from build123d import *

# Parameters (mm, degrees)
SKETCH1_R           = 20
SKETCH1_R_2         = 12
SKETCH1_R_3         = 2.5
SKETCH1_R_4         = 10
BOSS_EXTRUDE1_DEPTH = 3
BOSS_EXTRUDE2_START = 10
SKETCH1_3_R         = 12
SKETCH1_3_R_2       = 10
BOSS_EXTRUDE2_DEPTH = 10


with BuildPart() as part:
    # Sketch1 → Boss-Extrude1 (new body)
    # profile 1 of 2: a face of its own
    with BuildSketch(Plane(origin=(0, 0, 0), x_dir=(1, 0, 0), z_dir=(0, 1, 0))):
        with Locations(Location((0, 0, 0), (0, 0, 270))):
            Circle(SKETCH1_R)
        Circle(SKETCH1_R_2, mode=Mode.SUBTRACT)
        with Locations(Location((-12.990381057, -7.5, 0), (0, 0, 270))):
            Circle(SKETCH1_R_3, mode=Mode.SUBTRACT)
        with Locations(Location((12.990381057, -7.5, 0), (0, 0, 270))):
            Circle(SKETCH1_R_3, mode=Mode.SUBTRACT)
        with Locations(Location((0, 15, 0), (0, 0, 270))):
            Circle(SKETCH1_R_3, mode=Mode.SUBTRACT)
    # profile 2 of 2: a face of its own
    with BuildSketch(Plane(origin=(0, 0, 0), x_dir=(1, 0, 0), z_dir=(0, 1, 0))):
        Circle(SKETCH1_R_2)
        with Locations(Location((0, 0, 0), (0, 0, 270))):
            Circle(SKETCH1_R_4, mode=Mode.SUBTRACT)
    extrude(amount=-BOSS_EXTRUDE1_DEPTH)

    # Sketch1_3 → Boss-Extrude2 (add)
    with BuildSketch(Plane(origin=(0, 0, 0), x_dir=(1, 0, 0), z_dir=(0, 1, 0)).offset(BOSS_EXTRUDE2_START)):
        with Locations(Location((0, 0, 0), (0, 0, 270))):
            Circle(SKETCH1_3_R)
        with Locations(Location((0, 0, 0), (0, 0, 270))):
            Circle(SKETCH1_3_R_2, mode=Mode.SUBTRACT)
    extrude(amount=-BOSS_EXTRUDE2_DEPTH)


solid = part.part
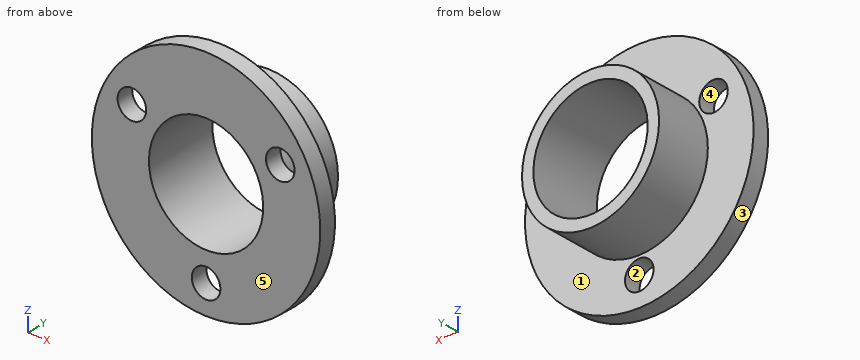
For this review, take the finished solid that the model builds, in its own axes (mm). Face numbers are marked on the shaded views. A direction names the side the tool comes from. Coordinates: 2 decimals unless noted, no trailing zeros. Loops run counter-clockwise (first coordinate to the right, second up) from the corner with the lowest first, then second, coordinate; pieces in that order, holes last. Notation, with made-up numbers: (69, -1) - (93, -1) arc R21 cw to (93, 18) - close; hole circle Ø10 at (79.25, 54). An arc over 180 degrees is marked (long way). Return JSON: item names as keys, results as strings.
Item 1: Mouldability with a two-part tool opening along Z and no side actions: class the marked faces 3, 4 and 5 as pulls with the +Z half, pulls with the -Z half, needs draft (parallel to the pull), parting line crosses it, or undercut.
Determined:
{"face 3": "parting line crosses it", "face 4": "undercut", "face 5": "needs draft"}
Item 2: For the marked faces 1 and 2, list the 3-axis set-ups (+Z, -Z, +X, -X, +Y, -Y) from which the entire face can be reached by the end or side of a thin tool; tool diameter is ignored.
Determined:
{"face 1": "+Y", "face 2": "+Y, -Y"}
Item 3: Take a section at B-B (z = 0). Give the boundary of the cut face in (x, y), then the cut area to 3 significant figures.
Determined:
{"outline": "(-20, -3) - (-10, -3) - (-10, 10) - (-12, 10) - (-12, 0) - (-20, 0) - close; (10, -3) - (20, -3) - (20, 0) - (12, 0) - (12, 10) - (10, 10) - close", "area": "100 mm2"}
Item 4: For line 1 (X direction, y = -1.2, z = 7.5); line 2 (X direction, y = 2.75, z = 0); line 3 (Y direction, x = -10, z = 9.5), list the stretches that pass through material, from the lowest coordinate up.
Determined:
{"line 1": "x = -18.54 to -15.49, -10.49 to -6.61, 6.61 to 10.49, 15.49 to 18.54", "line 2": "x = -12 to -10, 10 to 12", "line 3": "y = -3 to 0"}
Item 5: Take a section at C-C (z = 5.5). Give the boundary of the cut face in (x, y).
Determined:
{"outline": "(-19.23, -3) - (-14.49, -3) - (-14.49, 0) - (-19.23, 0) - close; (-11.49, -3) - (-8.35, -3) - (-8.35, 10) - (-10.67, 10) - (-10.67, 0) - (-11.49, 0) - close; (8.35, -3) - (11.49, -3) - (11.49, 0) - (10.67, 0) - (10.67, 10) - (8.35, 10) - close; (14.49, -3) - (19.23, -3) - (19.23, 0) - (14.49, 0) - close"}
Item 6: Insertion check: pin 1 (1 mm diameter, centred on y = 5.5, z = 5, fed in from +X); pin 2 (4 mm diameter, centred on x = -12.99, z = 7.5, fed in from -Y); pin 3 (5 mm diameter, centred on x = 10, y = 7, fed in from -Z); pin 4 (6 mm diameter, centred on y = 5, z = 0.5, fed in from +X). Each pin has a flat end and moves straight along its axis. Give the tip position at first contact, or say it passes through.
Determined:
{"pin 1": "stops at x = 11.12", "pin 2": "passes through", "pin 3": "stops at z = -9.37", "pin 4": "stops at x = 12"}
Item 7: Take a section at D-D (y = 1). Give the boundary of the cut face in (x, z), then the cut area to 3 significant figures.
Determined:
{"outline": "circle Ø24 at (0, 0); hole circle Ø20 at (0, 0)", "area": "138 mm2"}
Item 8: Take a section at A-A (x = 0). Give the boundary of the cut face in (y, z), then the cut area to 3 significant figures.
Determined:
{"outline": "(-3, -20) - (0, -20) - (0, -17.5) - (-3, -17.5) - close; (-3, -12.5) - (0, -12.5) - (0, -12) - (10, -12) - (10, -10) - (-3, -10) - close; (-3, 10) - (10, 10) - (10, 12) - (0, 12) - (0, 20) - (-3, 20) - close", "area": "85.0 mm2"}
